The model under review builds one solid part; all positions refer to its coordinate system, in mm. A direction names the side the tool comes from. Coordinates: 2 decimals unless noted, no trailing zeros. Loops run counter-clockwise (first coordinate to the right, second up) from the corner with the lowest first, then second, coordinate; pieces in that order, holes last. Notation, with made-up numbers: (69, -2) - (112, -2) arc R23 cw to (112, 32) - close; hole circle Ø8 at (-20.5, 39). An arc over 180 degrees is marked (long way). Answer in a Markdown table with one row per item. Add a question column.
(1) For line 1 along Y through (x, z) = (-4.25, 13.5); line 2 along Z through (x, y) = (-14, 1); line 3 along Y through (x, z) = (-3.25, 11), list the stretches that pass through material, from the lowest coordinate up.
(2) We need section B-B on y = 11. Write out the cut boundary in (x, z), plus the area to 3 significant figures.
(3) For P1, Ø3, axis at x = 0, y = 1, coming from the +Z side; P2, Ø6, axis at x = -5, y = 7, coming from the +Z side; P3, Ø2, axis at x = -10.5, y = 0.5, coming from the -Z side, all flat-tipped, find the tip position at first contact; note any pin that passes through.
(4) Mouldability with a two-part tool opening along Z and no side actions: class faces 6 (the flat face through (-6, 10.16, 14)), 7 (the flat face through (-8.349, 1, 7)), 8 (the flat face through (-11, 1, 16.802)) as +Z half, -Z half, draft (parallel to the pull), parting line (faces both ways), or undercut.
(5) Machinability: for faces 1 (the flat face through (-1.999, 1, 7)), 2 (the flat face through (-5, 1, 23.152)), 3 (the flat face through (-12, 1, 10.452)), 4 (the flat face through (1, 1, 16.802)), 5 (the flat face through (-5, 1.27, 14)), which of the approach directions +Z, -Z, +X, -X, +Y, -Y give a long, thin tool a straight path to every point of the face, cutting with its end or side? Answer none if there is none.
(6) We need section A-A on y = 8.25. Give the number of separate pieces and of enclosed holes in the cut face, plus the area to 3 significant figures.
from build123d import *

# Parameters (mm, degrees)
BODY_DEPTH        = 2.54
SKETCH2_R         = 1.905
LEGS_DEPTH        = 7.62
SKETCH4_R         = 1.905
SPRING_HOLE_DEPTH = 1.27
SKETCH5_R         = 10.040231571
FOOT_DEPTH        = 2.54
SKETCH6_R         = 2.54
FLAG_DEPTH        = 2.54
ROUNDITY_R        = 2.54


with BuildPart() as part:
    # Sketch1 → body (new body)
    with BuildSketch(Plane(origin=(0, 0, 0), x_dir=(1, 0, 0), z_dir=(0, 1, 0))):
        Polygon((-8.348684361, -10.452067183), (-8.348684361, -4.102067183), (-1.998684361, -4.102067183), (-1.998684361, -10.452067183), (4.351315639, -10.452067183), (4.351315639, -16.802067183), (-1.998684361, -16.802067183), (-1.998684361, -23.152067183), (-8.348684361, -23.152067183), (-8.348684361, -16.802067183), (-14.698684361, -16.802067183), (-14.698684361, -10.452067183), align=None)
    extrude(amount=BODY_DEPTH)

    # Sketch2 → legs (add)
    with BuildSketch(Plane(origin=(0, 2.54, 0), x_dir=(1, 0, 0), z_dir=(0, 1, 0))):
        with Locations(Location((-5.173684361, -7.277067183, 0), (0, 0, 90))):
            Circle(SKETCH2_R)
        with Locations(Location((1.176315639, -13.627067183, 0), (0, 0, 90))):
            Circle(SKETCH2_R)
        with Locations(Location((-5.173684361, -19.977067183, 0), (0, 0, 90))):
            Circle(SKETCH2_R)
        with Locations(Location((-11.523684361, -13.627067183, 0), (0, 0, 90))):
            Circle(SKETCH2_R)
    extrude(amount=LEGS_DEPTH)

    # Sketch4 → spring hole (cut)
    with BuildSketch(Plane(origin=(0, 2.54, 0), x_dir=(1, 0, 0), z_dir=(0, 1, 0))):
        with Locations(Location((-5.173684361, -13.627067183, 0), (0, 0, 270))):
            Circle(SKETCH4_R)
    extrude(amount=-SPRING_HOLE_DEPTH, mode=Mode.SUBTRACT)

    # Sketch5 → foot (add)
    with BuildSketch(Plane(origin=(0, 10.16, 0), x_dir=(1, 0, 0), z_dir=(0, 1, 0))):
        with Locations(Location((-5.173684361, -13.627067183, 0), (0, 0, 270))):
            Circle(SKETCH5_R)
    extrude(amount=FOOT_DEPTH)

    # Sketch6 → flag (add)
    with BuildSketch(Plane(origin=(0, 12.7, 0), x_dir=(1, 0, 0), z_dir=(0, 1, 0))):
        with Locations(Location((-5.173684361, -13.627067183, 0), (0, 0, 270))):
            Circle(SKETCH6_R)
    extrude(amount=FLAG_DEPTH)

    # roundity
    roundity_edges = [part.edges().sort_by_distance(p)[0] for p in [
        (-5.173684361, 10.16, 9.182067183),
        (1.176315639, 10.16, 15.532067183),
        (-5.173684361, 10.16, 21.882067183),
        (-11.523684361, 10.16, 15.532067183),
        (-5.173684361, 12.7, 11.087067183),
    ]]
    fillet(roundity_edges, radius=ROUNDITY_R - 0.0001)  # a hair under: the kernel refuses the full size


solid = part.part
Outcome:
| question | item | result |
|---|---|---|
| 1 | line 1 | 0 to 1.27, 10.16 to 15.24 |
| 1 | line 2 | 10.45 to 16.8 |
| 1 | line 3 | 0 to 2.54, 10.15 to 13.47 |
| 2 | outline | circle Ø20.08 at (-5.17, 13.63) |
| 2 | area | 317 mm² |
| 3 | P1 | z = 16.8 |
| 3 | P2 | z = 23.27 |
| 3 | P3 | z = 10.45 |
| 4 | face 6 | undercut |
| 4 | face 7 | draft |
| 4 | face 8 | +Z half |
| 5 | face 1 | -Z, +X, -Y |
| 5 | face 2 | +Z, +X, -X, -Y |
| 5 | face 3 | -Z, -X, -Y |
| 5 | face 4 | +Z, +X, -Y |
| 5 | face 5 | none |
| 6 | separate pieces | 4 |
| 6 | enclosed holes | 0 |
| 6 | area | 49.3 mm² |
